Geometry: see drawing. Coordinates: mm, zero at the bounding-box minimum. A direction names the side the tool comes from. Round coordinates to 2 decimals unless told otherwise and drop trailing zeros. Loops run counter-clockwise (first coordinate to the right, second up) from the corner with the lowest first, then second, coordinate; pieces in that order, holes last. Notation, with made-up numbers: (32.25, -12) -> (39.25, -12) arc R3 ccw to (39.25, -7) -> close; hole circle Ø7 at (51.5, -17). An arc over 180 degrees is marked (long way). Answer in a Markdown table with one row per item.
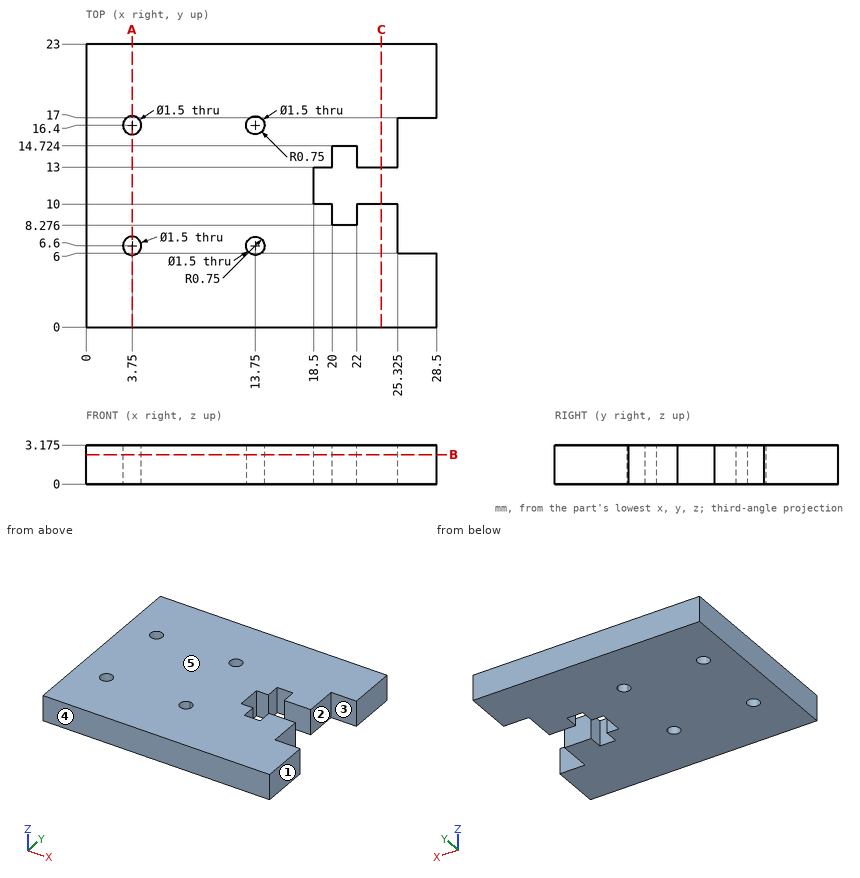
Item 1: Ray query, L1, parallel to Y at x = 3.75, z = 2.55; L2, parallel to X at y = 14.5, z = 2.95 (3 decimals); L3, parallel to X at y = 12, z = 0.2. Return the intervals inside material, ascending.
Ans:
| item | result |
|---|---|
| L1 | 0 to 5.85, 7.35 to 15.65, 17.15 to 23 |
| L2 | 0 to 20, 22 to 25.325 |
| L3 | 0 to 18.5 |
Item 2: Section query A-A, the plane x = 3.75. Output: boundary loops of the cut face in (y, z) (3 decimals).
Ans:
| item | result |
|---|---|
| outline | (0, 0) -> (5.85, 0) -> (5.85, 3.175) -> (0, 3.175) -> close; (7.35, 0) -> (15.65, 0) -> (15.65, 3.175) -> (7.35, 3.175) -> close; (17.15, 0) -> (23, 0) -> (23, 3.175) -> (17.15, 3.175) -> close |
Item 3: Mould query, pull axis Y, two halves, no side actions, for the marked faces 3, 4 and 5. Classes: released by +Y, released by -Y, zero draft, split by the parting line, or undercut.
Ans:
| item | result |
|---|---|
| face 3 | undercut |
| face 4 | released by -Y |
| face 5 | zero draft |
Item 4: Set-up query: the marked faces 1 and 2. Return all of +Z, -Z, +X, -X, +Y, -Y with unobstructed straight access to the full face (end or side cutting, diameter ignored); none if empty.
Ans:
| item | result |
|---|---|
| face 1 | +Z, -Z, +X, +Y, -Y |
| face 2 | +Z, -Z, +X |
Item 5: Section query B-B, the plane z = 2.4. State how many separate pieces and enclosed holes the cut face has, and give its area (3 significant figures).
Ans:
| item | result |
|---|---|
| separate pieces | 1 |
| enclosed holes | 4 |
| area | 586 mm2 |
Item 6: Section query C-C, the plane x = 24. Output: boundary loops of the cut face in (y, z) (3 decimals), and give its area (3 significant figures).
Ans:
| item | result |
|---|---|
| outline | (0, 0) -> (10, 0) -> (10, 3.175) -> (0, 3.175) -> close; (13, 0) -> (23, 0) -> (23, 3.175) -> (13, 3.175) -> close |
| area | 63.5 mm2 |
Item 7: First-contact query: P1, Ø0.9, axis at y = 14, z = 2, coming from the +X side (3 decimals); P2, Ø1.3, axis at x = 13.75, y = 6.6, coming from the +Z side; P3, Ø1.5, axis at y = 12, z = 2, coming from the +X side. Flat tips, straight axial feed; report the tip coordinate or a pass-through.
Ans:
| item | result |
|---|---|
| P1 | x = 25.325 |
| P2 | through |
| P3 | x = 18.5 |
